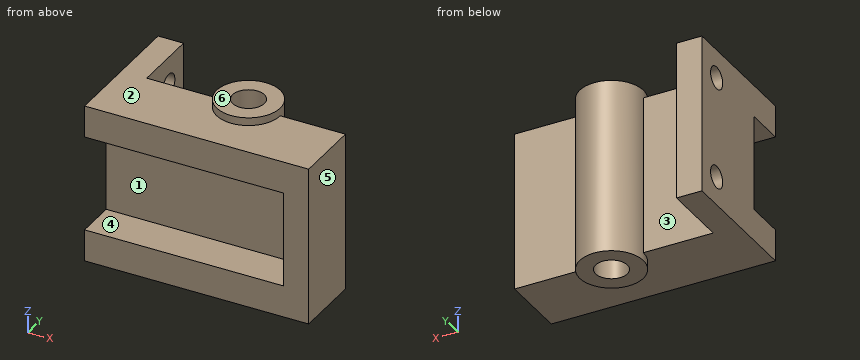
```python
from build123d import *

# Parameters (mm, degrees)
BOSS_EXTRUDE1_DEPTH      = 1270
BOSS_EXTRUDE1_DEPTH_BACK = 1270
BOSS_EXTRUDE2_DEPTH      = 1397
BOSS_EXTRUDE2_DEPTH_BACK = 1397
SKETCH1_3_R              = 508
SKETCH1_3_R_2            = 254
SKETCH2_W                = 1524
SKETCH2_H                = 635
CUT_EXTRUDE1_DEPTH       = 3175
SKETCH3_R                = 177.8
CUT_EXTRUDE2_DEPTH       = 508
SCALE1_SCALE             = 0.0393701


with BuildPart() as part:
    # Sketch1 → Boss-Extrude1 (new, two sides: drawn at the far end of the back side and taken through both)
    with BuildSketch(Plane.XY.offset(-BOSS_EXTRUDE1_DEPTH_BACK)):
        with BuildLine():
            Line((0, 2159), (0, 0))
            Line((0, 0), (3581.4, 0))
            Line((3581.4, 0), (3581.4, 1079.5))
            Line((3581.4, 1079.5), (2540, 1079.5))
            ThreePointArc((2540, 1079.5), (2032, 571.5), (1524, 1079.5))
            Line((1524, 1079.5), (406.4, 1079.5))
            Line((406.4, 1079.5), (406.4, 2159))
            Line((406.4, 2159), (0, 2159))
        make_face()
    extrude(amount=BOSS_EXTRUDE1_DEPTH + BOSS_EXTRUDE1_DEPTH_BACK)

    # Sketch1_3 → Boss-Extrude2 (add, two sides: drawn at the far end of the back side and taken through both)
    with BuildSketch(Plane.XY.offset(-BOSS_EXTRUDE2_DEPTH_BACK)):
        with Locations((2032, 1079.5)):
            Circle(SKETCH1_3_R)
        with Locations((2032, 1079.5)):
            Circle(SKETCH1_3_R_2, mode=Mode.SUBTRACT)
    extrude(amount=BOSS_EXTRUDE2_DEPTH + BOSS_EXTRUDE2_DEPTH_BACK)

    # Sketch2 → Cut-Extrude1 (cut)
    with BuildSketch(Plane.ZY):
        with Locations((0, 317.5)):
            Rectangle(SKETCH2_W, SKETCH2_H)
    extrude(amount=-CUT_EXTRUDE1_DEPTH, mode=Mode.SUBTRACT)

    # Sketch3 → Cut-Extrude2 (cut)
    with BuildSketch(Plane.ZY):
        with Locations(Location((-812.8, 1727.2, 0), (0, 0, 270))):
            Circle(SKETCH3_R)
        with Locations(Location((812.8, 1727.2, 0), (0, 0, 270))):
            Circle(SKETCH3_R)
    extrude(amount=-CUT_EXTRUDE2_DEPTH, mode=Mode.SUBTRACT)


with BuildPart() as part_1:
    # Scale1: scaled about (1689.519743013, 820.589305636, 0)
    add(part.part.scale(SCALE1_SCALE).moved(Location((1623.003181779, 788.282622614, 0))))


solid = part_1.part
```
Input: part model. Units: mm. Frame: model coordinates. Face numbers are marked on the shaded views. A direction names the side the tool comes from. Coordinates: 2 decimals unless noted, no trailing zeros. Order: outer loops, then holes, each group sorted by start corner. A loop starts at its lowest first (then second) coordinate and runs counter-clockwise, first axis right, second up. Notation, with made-up numbers: (84, 73) - (129, 73) arc R27 cw to (129, 98) - close; hole circle Ø8 at (-33.5, 62.25). An arc over 180 degrees is marked (long way). Return JSON: item names as keys, results as strings.
Q1. Ray query, probe 1 along Z at (x, y) = (1732, 812.5); probe 2 along Y at (x, z) = (1703, 27); probe 3 along X at (y, z) = (795, 22). Return the intervals inside material, ascending.
The answers:
{"probe 1": "z = -50 to -30, 30 to 50", "probe 2": "y = 813.28 to 820.78, 840.78 to 850.78", "probe 3": "x = 1748 to 1764"}
Q2. Cut plane A-A (z = -13). Return loops of the section in (x, y), then the cut area to 3 significant figures.
The answers:
{"outline": "(1623, 813.28) - (1748, 813.28) - (1748, 788.28) - (1764, 788.28) - (1764, 830.78) - (1723, 830.78) arc R20 ccw to (1683, 830.78) - (1639, 830.78) - (1639, 873.28) - (1623, 873.28) - close; hole circle Ø20 at (1703, 830.78)", "area": "3,860 mm2"}
Q3. Cut plane B-B (y = 846.5). Return loops of the section in (x, z).
The answers:
{"outline": "(1623, -50) - (1639, -50) - (1639, 50) - (1623, 50) - close; (1690.64, -55) - (1715.37, -55) - (1715.37, 55) - (1690.64, 55) - close"}
Q4. Cut plane D-D (z = -35.5). Return loops of the section in (x, y).
The answers:
{"outline": "(1623, 788.28) - (1764, 788.28) - (1764, 830.78) - (1723, 830.78) arc R20 ccw to (1683, 830.78) - (1639, 830.78) - (1639, 850.22) - (1623, 850.22) - close; (1623, 862.34) - (1639, 862.34) - (1639, 873.28) - (1623, 873.28) - close; hole circle Ø20 at (1703, 830.78)"}
Q5. Draft query along Z for the marked faces 4, 5 and 6. Return one class per face: +Z half, -Z half, draft (parallel to the pull), parting line (faces both ways), or undercut.
The answers:
{"face 4": "undercut", "face 5": "draft", "face 6": "+Z half"}
Q6. Cut plane C-C (x = 1663). Return loops of the section in (y, z).
The answers:
{"outline": "(788.28, -50) - (830.78, -50) - (830.78, 50) - (788.28, 50) - (788.28, 30) - (813.28, 30) - (813.28, -30) - (788.28, -30) - close"}
Q7. Access query for the marked faces 1, 2 and 3. Directions: +Z, -Z, +X, -X, +Y, -Y. A direction counts if a zero-diameter tool reaches every point of the face in a straight line with its end or side. Return the directions, or none.
The answers:
{"face 1": "-X, -Y", "face 2": "+Z, -Y", "face 3": "+Z, -Z, +Y"}
Q8. First-contact query: pin 1 (12.5 mm diameter, centred on y = 806.5, z = -12, fed in from -X); pin 2 (22.5 mm diameter, centred on y = 856.28, z = -32, fed in from +X); pin 3 (8 mm diameter, centred on x = 1703, y = 801, fed in from -Z). Flat tips, straight axial feed; report the tip coordinate or a pass-through.
The answers:
{"pin 1": "stops at x = 1748", "pin 2": "stops at x = 1717.04", "pin 3": "stops at z = -50"}
